Check sheet for the drawn part. Datum: minimum x, y, z corner. Units: mm. A direction names the side the tool comes from. Coordinates: 2 decimals unless noted, no trailing zeros. Write each loop counter-clockwise with the first axis right and the second up, starting at its lowest first coordinate (ties: lowest second). Pieces come first, ordered by that corner, then holes. Notation, with made-up numbers: M 18.5,53.5 L 50.5,53.5 A23 ccw 50.5,89.5 Z; hole C 58.25,55.5 d10. An arc over 180 degrees is marked long. Answer as CSV lines item,"result". Start each with the question number.
Q1. Sectioned sample at B-B, the plane z = 2.15. Record the cut outline in (x, y) (3 decimals).
Q2. Thickness scan on line 1 along Y through (x, z) = (3, 1); line 2 along X through (y, z) = (3.25, 2.4) (3 decimals); line 3 along X through (y, z) = (1.5, 0.3) (3 decimals). Record the ranges inside material, lowest first. Write a range as from..to.
Q3. Access from +Z, -Z, +X, -X, +Y, -Y to the whole of each face (thin tool, end or side, straight path). Record for the marked faces 1, 2 and 3.
Q4. Sectioned sample at A-A, the plane y = 2.5. Record the cut outline in (x, z) (3 decimals), then the cut area to 3 significant figures.
Q5. Sectioned sample at C-C, the plane x = 39. Record the cut outline in (y, z).
Q6. Depth check by flat-ended pin: pin 1 Ø1 at (x, z) = (6.5, 1) entering from +Y; pin 2 Ø1 at (y, z) = (5.5, 2) entering from +X; pin 3 Ø0.6 at (x, z) = (21, 1) entering from -Y. Enter the tip coordinate at first touch or a pass-through.
Q7. Sectioned sample at D-D, the plane x = 13.5. Record the cut outline in (y, z), then the cut area to 3 significant figures.
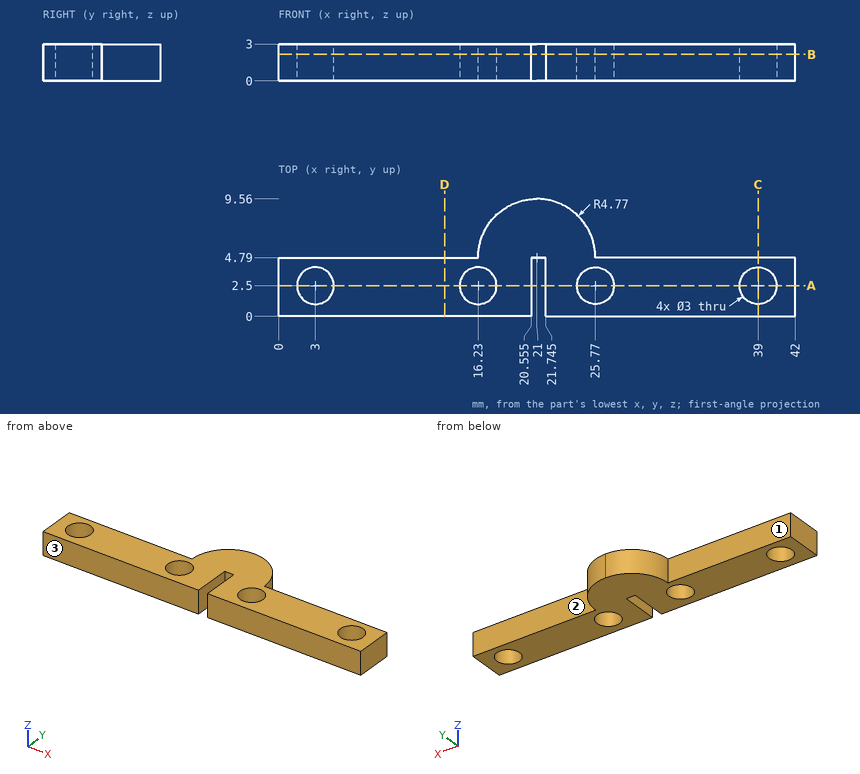
Output:
1,outline,"M 0,0 L 20.555,0 L 20.555,4.79 L 21.745,4.79 L 21.745,0 L 42,0 L 42,4.79 L 25.77,4.79 A4.77 ccw 16.23,4.79 L 0,4.79 Z; hole C 3,2.5 d3; hole C 16.23,2.5 d3; hole C 25.77,2.5 d3; hole C 39,2.5 d3"
2,line 1,"y = 0..1, 4..4.79"
2,line 2,"x = 0..1.701, 4.299..14.931, 17.529..20.555, 21.745..24.471, 27.069..37.701, 40.299..42"
2,line 3,"x = 0..1.882, 4.118..15.112, 17.348..20.555, 21.745..24.652, 26.888..37.882, 40.118..42"
3,face 1,"+Z, -Z, -X, +Y"
3,face 2,"+Z, -Z, +X, +Y"
3,face 3,"+Z, -Z, +X, -X, -Y"
4,outline,"M 0,0 L 1.5,0 L 1.5,3 L 0,3 Z; M 4.5,0 L 14.73,0 L 14.73,3 L 4.5,3 Z; M 17.73,0 L 20.555,0 L 20.555,3 L 17.73,3 Z; M 21.745,0 L 24.27,0 L 24.27,3 L 21.745,3 Z; M 27.27,0 L 37.5,0 L 37.5,3 L 27.27,3 Z; M 40.5,0 L 42,0 L 42,3 L 40.5,3 Z"
4,area,"86.4 mm^2"
5,outline,"M 0,0 L 1,0 L 1,3 L 0,3 Z; M 4,0 L 4.79,0 L 4.79,3 L 4,3 Z"
6,pin 1,"stops at y = 4.79"
6,pin 2,"stops at x = 25.77"
6,pin 3,"stops at y = 4.79"
7,outline,"M 0,0 L 4.79,0 L 4.79,3 L 0,3 Z"
7,area,"14.4 mm^2"
